Solid Edge part; units mm, degrees
sketch "Sketch1" plane through (0, 0, 0) normal (0, -1, 0) x (1, 0, 0)
  line L0 (-15, 15) -> (-15, -15)
  line L1 (-15, -15) -> (15, -15)
  line L2 (15, -15) -> (15, 15)
  line L3 (15, 15) -> (-15, 15)
  line L4 (-14, 14) -> (-14, -14)
  line L5 (-14, -14) -> (14, -14)
  line L6 (14, -14) -> (14, 14)
  line L7 (14, 14) -> (-14, 14)
extrude "Protrusion1" add sketch "Sketch1" along normal blind 160
sketch "Sketch2" plane through (-15, -100, 0) normal (-1, 0, 0) x (0, -1, 0)
  line L0 (-100, 15) -> (-17.5757, -15)
  line L1 (-100, -15) -> (-17.5757, -15)
  line L2 (-100, 15) -> (-100, -15)
extrude "ExtrudedCutout_1" cut sketch "Sketch2" against normal blind 853.4319
sketch "Sketch3" plane through (-15, -80, 0) normal (-1, 0, 0) x (0, -1, 0)
  line L0 (80, 15) -> (80, -15)
  line L1 (80, -15) -> (69.0809, -15)
  line L2 (80, 15) -> (69.0809, -15)
extrude "ExtrudedCutout_2" cut sketch "Sketch3" against normal blind 51.9593
fillet "Round_1" [suppressed]
Can you work these out from the model? Positions are in its coordinate system, mm. A direction names the side the tool comes from. Coordinates: 2 decimals unless noted, no trailing zeros. Write each loop counter-clockwise with the first axis right and the second up, starting at its lowest first coordinate (ties: lowest second). Pieces come first, ordered by that corner, then holes.
Q1. Imagine slicing it at B-B, the plane x = 2. List the corners of the cut face in (y, z) for me.
Results found:
outline: (-160, 15) - (-159.64, 14) - (-2.75, 14) - (0, 15) - close; (-149.44, -14) - (-149.08, -15) - (-82.42, -15) - (-79.68, -14) - close
Q2. Imagine slicing it at C-C, the plane z = -4.5. List the corners of the cut face in (x, y) for me, plus the area to 3 significant figures.
Results found:
outline: (-15, -152.9) - (-14, -152.9) - (-14, -53.58) - (-15, -53.58) - close; (14, -152.9) - (15, -152.9) - (15, -53.58) - (14, -53.58) - close
area: 199 mm2
Q3. If we mould it in two halves opening along X, with no side actions, what happens to faces 3 (the face through (0, -114, -14)), 4 (the face through (15, -97, 3)), 5 (the face through (14, -98, 0)), 6 (the face through (14.37, -37.97, 1.18))? For each: +X half, -X half, draft (parallel to the pull), parting line (faces both ways), or undercut.
Results found:
face 3: undercut
face 4: +X half
face 5: undercut
face 6: draft
Q4. Please list where these lines run through material, in increasing order: L1, parallel to Z at x = 2, y = -143; L2, parallel to Z at x = -9.5, y = -26.
Results found:
L1: z = -15 to -14, 14 to 15
L2: z = 14 to 15
Q5. Which directions (+Z, -Z, +X, -X, +Y, -Y) give clear straight access to the entire face, cutting with the end or side of a thin tool? Please do faces 1 (the face through (-15, -97, 4)), 2 (the face through (-14, -98, 0)).
Results found:
face 1: +Z, -Z, -X, +Y, -Y
face 2: +Y, -Y
Q6. For P1, Ø5, axis at x = -4, z = 9.5, coming from the +Y side; P2, Ø2, axis at x = 2.5, y = -18.5, coming from the -Z side, each with a flat end and sliding along its axis, tell me the tip position at first contact or that it passes through.
Results found:
P1: passes through
P2: stops at z = 14
Q7. Imagine slicing it at A-A, the plane y = -117.5. List the corners of the cut face in (x, z) for me.
Results found:
outline: (-15, -15) - (15, -15) - (15, 15) - (-15, 15) - close; hole (-14, -14) - (14, -14) - (14, 14) - (-14, 14) - close
Q8. Imagine slicing it at D-D, the plane y = -18.5. List the corners of the cut face in (x, z) for me.
Results found:
outline: (-15, 8.27) - (-14, 8.27) - (-14, 14) - (14, 14) - (14, 8.27) - (15, 8.27) - (15, 15) - (-15, 15) - close
